from build123d import *

# Parameters (mm, degrees)
F0_W     = 121.1435347795
F0_H     = 55.9340305626
F0_R     = 14.2505593298
F1_DEPTH = 7.3
F2_W     = 10
F2_H     = 55.9340305626
F3_DEPTH = 2


with BuildPart() as f1:
    # F0 (on Top) → F1 (new body)
    with BuildSketch(Plane.XY):
        Rectangle(F0_W, F0_H)
        Circle(F0_R, mode=Mode.SUBTRACT)
    extrude(amount=F1_DEPTH)

    # F2 (on face) → F3 (cut)
    with BuildSketch(Plane.XY.offset(7.3)):
        with BuildLine():
            Line((3.5, 27.9670152813), (-3.5, 27.9670152813))
            Line((-3.5, 27.9670152813), (-3.5, 13.8140667876))
            ThreePointArc((-3.5, 13.8140667876), (0, 14.2505593298), (3.5, 13.8140667876))
            Line((3.5, 13.8140667876), (3.5, 27.9670152813))
        make_face()
        with BuildLine():
            Line((-3.5, -13.8140667876), (-3.5, -27.9670152813))
            Line((-3.5, -27.9670152813), (3.5, -27.9670152813))
            Line((3.5, -27.9670152813), (3.5, -13.8140667876))
            ThreePointArc((3.5, -13.8140667876), (0, -14.2505593298), (-3.5, -13.8140667876))
        make_face()
        with Locations((-45.2155907452, 0)):
            Rectangle(F2_W, F2_H)
    extrude(amount=-F3_DEPTH, mode=Mode.SUBTRACT)


solid = f1.part
Verification items for the finished model (mm, model axes). A direction names the side the tool comes from. Give positions to 0.01 mm unless a question says otherwise; leave off trailing zeros. Write each loop counter-clockwise with the first axis right and the second up, starting at its lowest first coordinate (ties: lowest second). Pieces come first, ordered by that corner, then holes.
(1) Material ranges on line 1 (X direction, y = -21, z = 5.75); line 2 (Y direction, x = 0, z = 4.25); line 3 (X direction, y = 0, z = 4), recorded low to high.
(2) Cross-section at D-D (y = -22.5). Enter the section's corners in (x, z), plus the area to 3 significant figures.
(3) Mould release check, pull along X, two halves, no side actions. Record for faces 3 (the face through (0, -21, 5.3)), 4 (the face through (-60.572, 0, 4)), 5 (the face through (-14, 7, 0)): +X half, -X half, draft (parallel to the pull), parting line (faces both ways), or undercut.
(4) Cross-section at B-B (y = 0). Enter the section's corners in (x, z).
(5) Gauge pin test, flat ends, axial feed: pin 1 (11 mm diameter, centred on x = -45.5, y = 7.5, fed in from +Z); pin 2 (5.5 mm diameter, centred on x = -0.5, y = -22.5, fed in from +Z). Record the tip position at first contact, or that the pin passes through.
(6) Access from +Z, -Z, +X, -X, +Y, -Y to the whole of each face (thin tool, end or side, straight path). Record for faces 1 (the face through (0, 21, 5.3)), 2 (the face through (-1, -27.967, 4)).
(7) Cross-section at C-C (z = 3). Enter the section's corners in (x, y), plus the area to 3 significant figures.
(8) Cross-section at A-A (x = 0). Enter the section's corners in (y, z), plus the area to 3 significant figures.
Worked out:
1. line 1: x = -60.57 to -50.22, -40.22 to -3.5, 3.5 to 60.57
1. line 2: y = -27.97 to -14.25, 14.25 to 27.97
1. line 3: x = -60.57 to -14.25, 14.25 to 60.57
2. outline: (-60.57, 0) - (60.57, 0) - (60.57, 7.3) - (3.5, 7.3) - (3.5, 5.3) - (-3.5, 5.3) - (-3.5, 7.3) - (-40.22, 7.3) - (-40.22, 5.3) - (-50.22, 5.3) - (-50.22, 7.3) - (-60.57, 7.3) - close
2. area: 850 mm2
3. face 3: undercut
3. face 4: -X half
3. face 5: draft
4. outline: (-60.57, 0) - (-14.25, 0) - (-14.25, 7.3) - (-40.22, 7.3) - (-40.22, 5.3) - (-50.22, 5.3) - (-50.22, 7.3) - (-60.57, 7.3) - close; (14.25, 0) - (60.57, 0) - (60.57, 7.3) - (14.25, 7.3) - close
5. pin 1: stops at z = 7.3
5. pin 2: stops at z = 5.3
6. face 1: +Z, +Y, -Y
6. face 2: +Z, -Z, +X, -X, -Y
7. outline: (-60.57, -27.97) - (60.57, -27.97) - (60.57, 27.97) - (-60.57, 27.97) - close; hole circle Ø28.5 at (0, 0)
7. area: 6,140 mm2
8. outline: (-27.97, 0) - (-14.25, 0) - (-14.25, 5.3) - (-27.97, 5.3) - close; (14.25, 0) - (27.97, 0) - (27.97, 5.3) - (14.25, 5.3) - close
8. area: 145 mm2
